Check sheet for the modelled part. Datum: model origin and axes. Units: mm. Face numbers are marked on the shaded views. A direction names the side the tool comes from. Coordinates: 2 decimals unless noted, no trailing zeros. Loops run counter-clockwise (first coordinate to the right, second up) from the corner with the lowest first, then second, coordinate; pieces in that order, holes last. Notation, with made-up numbers: M 14.5,81.5 L 45.5,81.5 A9 ccw 45.5,97.5 Z; hole C -33,-30.75 d1. An arc over 180 degrees is marked long. Use CSV: the item, a comma, the result in double quotes. Start each with the question number.
(1) Scan lines: line 1 (Y direction, x = 20, z = 23) (3 decimals); line 2 (Y direction, x = 16, z = 15) (3 decimals); line 3 (X direction, y = -3, z = 15) (3 decimals). Record each from-to range of solid material in increasing order.
(2) Section check A-A on x = 10.5. Record the cut outline in (y, z) (3 decimals), and give its area (3 significant figures).
(3) Section check B-B on y = -30. Record the cut outline in (x, z) (3 decimals).
(4) Draft check along X on the marked faces 4, 5 and 6. Enter one of: pulls with the +X half, pulls with the -X half, needs draft (parallel to the pull), parting line crosses it, or undercut.
(5) Set-up check for the marked faces 1, 2 and 3: record each of +Z, -Z, +X, -X, +Y, -Y from which the full face is reachable in a straight line by a thin tool's end or side.
(6) Section check D-D on y = 6. Record the cut outline in (x, z) (3 decimals), and give its area (3 significant figures).
(7) Section check C-C on z = 9.6. Give the number of separate pieces and of enclosed holes in the cut face, and give its area (3 significant figures).
(8) Go/stop test with flat-tipped pins: pin 1 Ø0.9 at (y, z) = (18.5, 1.5) entering from +X; pin 2 Ø5 at (x, y) = (13, 10.5) entering from +Z; pin 3 Ø3 at (x, z) = (55.5, 19) entering from +Y. Record where each tip stops, or that it passes through.
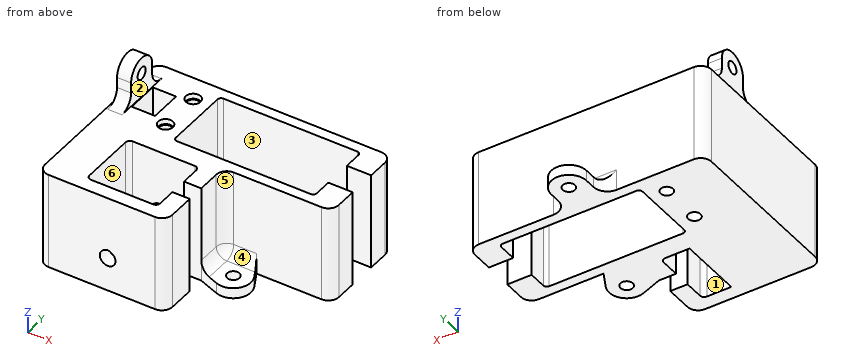
from build123d import *

# Parameters (mm, degrees)
SKETCH042_R     = 1.75
SKETCH042_W     = 6.65
SKETCH042_H     = 9.15
PAD015_DEPTH    = 27.5
SKETCH055_W     = 6.65
SKETCH055_H     = 9.15
SKETCH055_W_2   = 12
SKETCH055_H_2   = 18.15
PAD023_DEPTH    = 5
SKETCH056_R     = 1.75
PAD024_DEPTH    = 4
SKETCH057_R     = 1.75
PAD025_DEPTH    = 3
POCKET028_DEPTH = 13.5
SKETCH059_R     = 2.1
POCKET029_DEPTH = 1.5
FILLET_R        = 3


with BuildPart() as part:
    # Sketch042 → Pad015 (new body)
    with BuildSketch(Plane(origin=(0, 0, 0), x_dir=(-1, 0, 0), z_dir=(0, 0, -1))):
        with BuildLine():
            Line((-28.5, -38), (1.8, -38))
            ThreePointArc((1.8, -38), (3.9213203436, -37.1213203436), (4.8, -35))
            Line((4.8, -35), (4.8, 10))
            ThreePointArc((4.8, 10), (3.9213203436, 12.1213203436), (1.8, 13))
            Line((1.8, 13), (-59.5, 13))
            ThreePointArc((-59.5, 13), (-61.6213203436, 12.1213203436), (-62.5, 10))
            Line((-62.5, 10), (-62.5, 4))
            Line((-62.5, 4), (-55.575, 4))
            Line((-55.575, 9.075), (-55.575, 4))
            ThreePointArc((-54.575, 10.075), (-55.2821067812, 9.7821067812), (-55.575, 9.075))
            Line((-16.425, 10.075), (-54.575, 10.075))
            ThreePointArc((-15.425, 9.075), (-15.7178932188, 9.7821067812), (-16.425, 10.075))
            Line((-15.425, -9.075), (-15.425, 9.075))
            ThreePointArc((-16.425, -10.075), (-15.7178932188, -9.7821067812), (-15.425, -9.075))
            Line((-54.575, -10.075), (-16.425, -10.075))
            ThreePointArc((-55.575, -9.075), (-55.2821067812, -9.7821067812), (-54.575, -10.075))
            Line((-55.575, -4), (-55.575, -9.075))
            Line((-62.5, -4), (-55.575, -4))
            Line((-62.5, -4), (-62.5, -10))
            ThreePointArc((-62.5, -10), (-61.6213203436, -12.1213203436), (-59.5, -13))
            Line((-59.5, -13), (-34.5, -13))
            ThreePointArc((-31.5, -16), (-32.3786796564, -13.8786796564), (-34.5, -13))
            Line((-31.5, -16), (-31.5, -22.5))
            Line((-26.575, -22.5), (-31.5, -22.5))
            Line((-26.575, -17.125), (-26.575, -22.5))
            ThreePointArc((-25.375, -15.925), (-26.2235281374, -16.2764718626), (-26.575, -17.125))
            Line((-7.625, -15.925), (-25.375, -15.925))
            ThreePointArc((-6.425, -17.125), (-6.7764718626, -16.2764718626), (-7.625, -15.925))
            Line((-6.425, -32.875), (-6.425, -17.125))
            ThreePointArc((-7.625, -34.075), (-6.7764718626, -33.7235281374), (-6.425, -32.875))
            Line((-25.375, -34.075), (-7.625, -34.075))
            ThreePointArc((-26.575, -32.875), (-26.2235281374, -33.7235281374), (-25.375, -34.075))
            Line((-26.575, -27.5), (-26.575, -32.875))
            Line((-31.5, -27.5), (-26.575, -27.5))
            Line((-31.5, -27.5), (-31.5, -35))
            ThreePointArc((-31.5, -35), (-30.6213203436, -37.1213203436), (-28.5, -38))
        make_face()
        with Locations((-10.5, 6)):
            Circle(SKETCH042_R, mode=Mode.SUBTRACT)
        with Locations((-10.5, -6)):
            Circle(SKETCH042_R, mode=Mode.SUBTRACT)
        with Locations((-3.25, 0)):
            Rectangle(SKETCH042_W, SKETCH042_H, mode=Mode.SUBTRACT)
    extrude(amount=-PAD015_DEPTH)

    # Sketch055 → Pad023 (join)
    with BuildSketch(Plane(origin=(0, 0, 0), x_dir=(-1, 0, 0), z_dir=(0, 0, -1))):
        with Locations((-3.25, 0)):
            Rectangle(SKETCH055_W, SKETCH055_H)
        with Locations((-12.425, -25)):
            Rectangle(SKETCH055_W_2, SKETCH055_H_2)
    extrude(amount=-PAD023_DEPTH)

    # Sketch056 → Pad024 (join)
    with BuildSketch(Plane.YZ.offset(-0.25)):
        with BuildLine():
            Line((-8.575, 27.5), (8.575, 27.5))
            ThreePointArc((4.575, 31.5), (5.7465728753, 28.6715728753), (8.575, 27.5))
            Line((4.575, 31.5), (4.575, 34.5))
            ThreePointArc((4.575, 34.5), (0, 39.075), (-4.575, 34.5))
            Line((-4.575, 34.5), (-4.575, 31.5))
            ThreePointArc((-8.575, 27.5), (-5.7465728753, 28.6715728753), (-4.575, 31.5))
        make_face()
        with Locations((0, 34.5)):
            Circle(SKETCH056_R, mode=Mode.SUBTRACT)
    extrude(amount=-PAD024_DEPTH)

    # Sketch057 → Pad025 (join)
    with BuildSketch(Plane.XY):
        with BuildLine():
            ThreePointArc((34.5, -13), (32.3786796564, -13.8786796564), (31.5, -16))
            Line((31.5, -16), (31.5, -22.5))
            Line((31.5, -22.5), (37.2247448714, -24.6742346142))
            ThreePointArc((37.2247448714, -24.6742346142), (42.7342236735, -23.3249922641), (43.4377847505, -17.6965099287))
            Line((43.4377847505, -17.6965099287), (41, -13))
            Line((34.5, -13), (41, -13))
        make_face()
        with Locations((39, -20)):
            Circle(SKETCH057_R, mode=Mode.SUBTRACT)
        with BuildLine():
            Line((20.2, 13), (38.2, 13))
            ThreePointArc((34.2, 17), (35.3715728753, 14.1715728753), (38.2, 13))
            Line((34.2, 17), (34.2, 20))
            ThreePointArc((34.2, 20), (29.2, 25), (24.2, 20))
            Line((24.2, 17), (24.2, 20))
            ThreePointArc((20.2, 13), (23.0284271247, 14.1715728753), (24.2, 17))
        make_face()
        with Locations((29.2, 20)):
            Circle(SKETCH057_R, mode=Mode.SUBTRACT)
    extrude(amount=PAD025_DEPTH)

    # Sketch058 → Pocket028 (cut, symmetric)
    with BuildSketch(Plane(origin=(15, -25, 9.6), x_dir=(1, 0, 0), z_dir=(0, -1, 0))):
        with BuildLine():
            ThreePointArc((-0.9245936608, 2.05125), (0, -2.25), (0.9245936608, 2.05125))
            ThreePointArc((0.9245936608, 2.05125), (0, 2.4), (-0.9245936608, 2.05125))
        make_face()
    extrude(amount=POCKET028_DEPTH, both=True, mode=Mode.SUBTRACT)

    # Sketch059 (on Face5 of Pocket028) → Pocket029 (cut)
    with BuildSketch(Plane.XY.offset(27.5)):
        with Locations((10.5, 6)):
            Circle(SKETCH059_R)
        with Locations((10.5, -6)):
            Circle(SKETCH059_R)
    extrude(amount=-POCKET029_DEPTH, mode=Mode.SUBTRACT)

    # Fillet
    fillet_edges = [part.edges().sort_by_distance(p)[0] for p in [
        (32.37868, -13.87868, 3),
        (29.2, 13, 3),
    ]]
    fillet(fillet_edges, radius=FILLET_R)


solid = part.part
Outcome:
1,line 1,"y = -38 to -34.075, -15.925 to -10.075, 10.075 to 13"
1,line 2,"y = -38 to -34.075, -15.925 to -9.98, 9.98 to 13"
1,line 3,"x = -4.8 to -0.075, 6.575 to 15.425"
2,outline,"M -38,0 L -7.75,0 L -7.75,26 L -8.1,26 L -8.1,27.5 L -15.925,27.5 L -15.925,5 L -34.075,5 L -34.075,27.5 L -38,27.5 Z; M -4.25,0 L 4.25,0 L 4.25,26 L 3.9,26 L 3.9,27.5 L -3.9,27.5 L -3.9,26 L -4.25,26 Z; M 7.75,0 L 13,0 L 13,27.5 L 8.1,27.5 L 8.1,26 L 7.75,26 Z"
2,area,"800 mm²"
3,outline,"M -4.8,0 L 18.425,0 L 18.425,5 L 6.425,5 L 6.425,27.5 L -4.8,27.5 Z; M 26.575,0 L 31.5,0 L 31.5,27.5 L 26.575,27.5 Z"
4,face 4,"needs draft"
4,face 5,"pulls with the +X half"
4,face 6,"undercut"
5,face 1,"+Z"
5,face 2,"+Z, +X, +Y, -Y"
5,face 3,"+Z, -Z"
6,outline,"M -4.8,0 L 8.75,0 L 8.75,26 L 8.4,26 L 8.4,27.5 L -0.25,27.5 L -0.25,28.439 L -4.25,28.439 L -4.25,27.5 L -4.8,27.5 Z; M 12.25,0 L 15.425,0 L 15.425,27.5 L 12.6,27.5 L 12.6,26 L 12.25,26 Z; M 55.575,0 L 62.5,0 L 62.5,27.5 L 55.575,27.5 Z"
6,area,"653 mm²"
7,separate pieces,"2"
7,enclosed holes,"3"
7,area,"1,280 mm²"
8,pin 1,"stops at x = 34.2"
8,pin 2,"stops at z = 27.5"
8,pin 3,"stops at y = 13"
